```python
from build123d import *

# Parameters (mm, degrees)
BOSS_EXTRU_1_DEPTH      = 5
ESQUISSE2_W             = 20
ESQUISSE2_H             = 20
ENL_V_MAT_EXTRU_1_DEPTH = 5


with BuildPart() as part:
    # Esquisse1 → Boss.-Extru.1 (new body)
    with BuildSketch(Plane.XY):
        Polygon((-112.248737342, -130), (-87.5, -154.748737342), (87.5, -154.748737342), (112.248737342, -130), (112.248737342, 130), (87.5, 154.748737342), (-87.5, 154.748737342), (-112.248737342, 130), align=None)
    extrude(amount=BOSS_EXTRU_1_DEPTH)

    # Esquisse2 → Enlèv. mat.-Extru.1 (cut)
    with BuildSketch(Plane.XY.offset(5)):
        with Locations((-65, 131.748737342)):
            Rectangle(ESQUISSE2_W, ESQUISSE2_H)
        with Locations((-65, -131.748737342)):
            Rectangle(ESQUISSE2_W, ESQUISSE2_H)
        with Locations((65, -131.748737342)):
            Rectangle(ESQUISSE2_W, ESQUISSE2_H)
        with Locations((65, 131.748737342)):
            Rectangle(ESQUISSE2_W, ESQUISSE2_H)
    extrude(amount=-ENL_V_MAT_EXTRU_1_DEPTH, mode=Mode.SUBTRACT)


solid = part.part
```
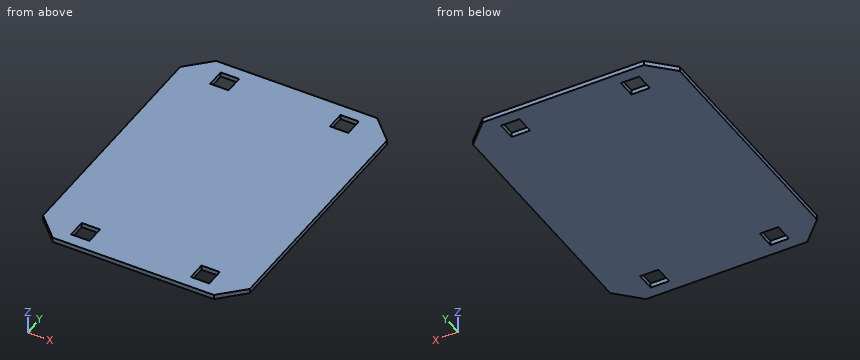
Model file for the job. Use its own axes, mm. Coordinates: 2 decimals unless noted, no trailing zeros. Order: outer loops, then holes, each group sorted by start corner. A loop starts at its lowest first (then second) coordinate and runs counter-clockwise, first axis right, second up. Notation, with made-up numbers: (42, 26) -> (74, 26) arc R28 cw to (74, 59) -> close; hole circle Ø10 at (40, -4.5). An arc over 180 degrees is marked (long way). Answer as a JSON object with one key per item and string values. Group by question number.
1) Flat gauge pin, fed straight in: pin 1 (2.5 mm diameter, centred on y = 131.5, z = 2, fed in from -X). Where does the tip first touch, or does it go through?
2) Drill centre lines: L1, parallel to Y at x = 73.5, z = 3.5; L2, parallel to Y at x = 103, z = 3.45; L3, parallel to Y at x = 89, z = 3.3. Where is each one in solid material? Low to high.
3) Cut at A-A, the plane z = 4.2. Write the cut outline in (x, y).
4) Cut at B-B, the plane x = -61.5. Write the cut outline in (y, z), then the cut area to 3 significant figures.
Check values:
{
 "1": {"pin 1": "stops at x = -112"},
 "2": {"L1": "y = -154.75 to -141.75, -121.75 to 121.75, 141.75 to 154.75", "L2": "y = -139.25 to 139.25", "L3": "y = -153.25 to 153.25"},
 "3": {"outline": "(-112.25, -130) -> (-87.5, -154.75) -> (87.5, -154.75) -> (112.25, -130) -> (112.25, 130) -> (87.5, 154.75) -> (-87.5, 154.75) -> (-112.25, 130) -> close; hole (-75, -141.75) -> (-55, -141.75) -> (-55, -121.75) -> (-75, -121.75) -> close; hole (-75, 121.75) -> (-55, 121.75) -> (-55, 141.75) -> (-75, 141.75) -> close; hole (55, -141.75) -> (75, -141.75) -> (75, -121.75) -> (55, -121.75) -> close; hole (55, 121.75) -> (75, 121.75) -> (75, 141.75) -> (55, 141.75) -> close"},
 "4": {"outline": "(-154.75, 0) -> (-141.75, 0) -> (-141.75, 5) -> (-154.75, 5) -> close; (-121.75, 0) -> (121.75, 0) -> (121.75, 5) -> (-121.75, 5) -> close; (141.75, 0) -> (154.75, 0) -> (154.75, 5) -> (141.75, 5) -> close", "area": "1,350 mm²"}
}
